For this review, take the finished solid that the model builds, in its own axes (mm). A direction names the side the tool comes from. Give positions to 0.01 mm unless a question says otherwise; leave off trailing zeros. Write each loop counter-clockwise with the first axis right and the second up, starting at its lowest first coordinate (ties: lowest second). Pieces come first, ordered by that corner, then holes. Notation, with made-up numbers: (54, -25) -> (79, -25) arc R29 ccw to (79, 3) -> close; hole circle Ø5 at (17.5, -40). An arc over 180 degrees is marked (long way). Return JSON: item names as keys, results as strings.
from build123d import *

# Parameters (mm, degrees)
F1_DEPTH = 19
F2_R     = 4
F3_DEPTH = 120.001
F4_R     = 9.49999


# Not quite as in the source:
# - a fillet or chamfer is up to 0.001 mm smaller than in the source, because OpenCascade refuses the exact size


with BuildPart() as f1:
    # F0 (on Front) → F1 (new body)
    with BuildSketch(Plane.XZ):
        Polygon((-45, -50), (45, -50), (45, -28), (75, -28), (75, 50), (-75, 50), (-75, -28), (-45, -28), align=None)
    extrude(amount=F1_DEPTH)

    # F2 (on face) → F3 (cut, through all)
    with BuildSketch(Plane(origin=(-45, 0, 0), x_dir=(0, -1, 0), z_dir=(-1, 0, 0))):
        with Locations((9.5, -40.5)):
            Circle(F2_R)
    extrude(amount=-F3_DEPTH, mode=Mode.SUBTRACT)

    # F4 (radius 9.5 in the source; OpenCascade refuses exactly that, so slightly less here)
    f4_edges = [f1.edges().sort_by_distance(p)[0] for p in [
        (0, 0, -50),
        (0, -19, -50),
    ]]
    fillet(f4_edges, radius=F4_R)


solid = f1.part
1. For pin 1 (5 mm diameter, centred on x = 50, z = 8.5, fed in from +Y); pin 2 (3 mm diameter, centred on y = -12.5, z = -30, fed in from +X); pin 3 (9.5 mm diameter, centred on x = 67, y = -13, fed in from -Z), all flat-tipped, find the tip position at first contact; note any pin that passes through.
Results found:
{"pin 1": "stops at y = 0", "pin 2": "stops at x = 45", "pin 3": "stops at z = -28"}
2. To check wall thickness, follow probe 1 along Z at (x, y) = (25, -9.5); probe 2 along Y at (x, z) = (-20, -40); probe 3 along X at (y, z) = (-2, -46). State the ranges of each line that lie inside material, in increasing order.
Results found:
{"probe 1": "z = -50 to -44.5, -36.5 to 50", "probe 2": "y = -19 to -13.47, -5.53 to 0", "probe 3": "x = -45 to 45"}
3. Add section D-D, the plane x = 60.5. State the section outline as (y, z) points, plus the area to 3 significant figures.
Results found:
{"outline": "(-19, -28) -> (0, -28) -> (0, 50) -> (-19, 50) -> close", "area": "1,480 mm²"}
4. The part is to be moulded in two halves that separate along Y. For faces 1 (the cylindrical face through (-0.63, -8.979, -36.534)), 2 (the flat face through (-1, -19, 5)), 3 (the flat face through (-1, 0, 5)), 4 (the flat face through (60, -9, -28)), say which applies: +Y half, -Y half, draft (parallel to the pull), parting line (faces both ways), or undercut.
Results found:
{"face 1": "undercut", "face 2": "-Y half", "face 3": "+Y half", "face 4": "draft"}
5. Add section B-B, the plane y = -8. State the section outline as (x, z) points, plus the area to 3 significant figures.
Results found:
{"outline": "(-75, -28) -> (-45, -28) -> (-45, -36.79) -> (45, -36.79) -> (45, -28) -> (75, -28) -> (75, 50) -> (-75, 50) -> close; (-45, -49.88) -> (45, -49.88) -> (45, -44.21) -> (-45, -44.21) -> close", "area": "13,000 mm²"}
6. For faces 5 (the flat face through (45, -7, -37)), 6 (the cylindrical face through (0.63, -16.143, -47.291)), 7 (the flat face through (-45, -9, -36)), list the 3-axis set-ups (+Z, -Z, +X, -X, +Y, -Y) from which the entire face can be reached by the end or side of a thin tool; tool diameter is ignored.
Results found:
{"face 5": "-Z, +X, +Y, -Y", "face 6": "-Z, +X, -X, -Y", "face 7": "-Z, -X, +Y, -Y"}
7. Add section C-C, the plane z = -42. State the section outline as (x, y) points, plus the area to 3 significant figures.
Results found:
{"outline": "(-45, -18.88) -> (45, -18.88) -> (45, -13.21) -> (-45, -13.21) -> close; (-45, -5.79) -> (45, -5.79) -> (45, -0.12) -> (-45, -0.12) -> close", "area": "1,020 mm²"}
